Design review of the part built by this model. Coordinates are the model's own, in mm. A direction names the side the tool comes from. Round coordinates to 2 decimals unless told otherwise and drop trailing zeros. Write each loop counter-clockwise with the first axis right and the second up, starting at its lowest first coordinate (ties: lowest second). Pieces come first, ordered by that corner, then holes.
from build123d import *

# Parameters (mm, degrees)
F1_DEPTH = 4.064
F0_W     = 4.064
F0_H     = 4.064
F2_DEPTH = 4.064


# Not quite as in the source:
# - a feature names something its author has since deleted; it is built from what else it names


with BuildPart() as f1:
    # F0 (on Top) → F1 (new body)
    with BuildSketch(Plane.XY):
        Polygon((31.75, 12.7), (31.75, 25.4), (-31.75, 25.4), (-31.75, 12.7), (-27.686, 12.7), (-27.686, -12.7), (-31.75, -12.7), (-31.75, -25.4), (-25.4, -25.4), (-25.4, -21.336), (25.4, -21.336), (25.4, -25.4), (31.75, -25.4), (31.75, -12.7), (27.686, -12.7), (27.686, 12.7), align=None)
    extrude(amount=F1_DEPTH)

    # F0 (on Top) → F2 (join)
    with BuildSketch(Plane.XY):
        Polygon((21.336, -25.4), (25.4, -25.4), (25.4, -21.336), (-25.4, -21.336), (-25.4, -25.4), (-21.336, -25.4), align=None)
        with Locations((23.368, -27.432)):
            Rectangle(F0_W, F0_H)
        with Locations((-23.368, -27.432)):
            Rectangle(F0_W, F0_H)
        Polygon((31.75, 12.7), (31.75, 25.4), (-31.75, 25.4), (-31.75, 12.7), (-27.686, 12.7), (-27.686, -12.7), (-31.75, -12.7), (-31.75, -25.4), (-25.4, -25.4), (-25.4, -21.336), (25.4, -21.336), (25.4, -25.4), (31.75, -25.4), (31.75, -12.7), (27.686, -12.7), (27.686, 12.7), align=None)
    extrude(amount=F2_DEPTH)


solid = f1.part
1) Add section B-B on x = -12.5. State the section outline as (y, z) points, and give its area (3 significant figures).
2) The part is to be moulded in two halves that separate along Y. For faces 1 (the face through (0, -2, 4.064)), 2 (the face through (30, -12.7, 2)), 3 (the face through (-23, -29.464, 2)), say which applies: pulls with the +Y half, pulls with the -Y half, needs draft (parallel to the pull), parting line crosses it, or undercut.
3) For line 1 along Y through (x, z) = (-26.5, 1.75); line 2 along Y through (x, z) = (-28, 1.2); line 3 along X through (y, z) = (-8, 2.55), list the stretches that pass through material, from the lowest coordinate up.
4) For P1, Ø2, axis at x = 30, z = 2.5, coming from the -Y side; P2, Ø1.2, axis at y = -27.5, z = 1.5, coming from the -X side; P3, Ø1.2, axis at y = -27.5, z = 3, coming from the +X side, all flat-tipped, find the tip position at first contact; note any pin that passes through.
5) Add section A-A on z = 2.2. State the section outline as (x, y) points.
6) Add section C-C on y = -1. State the section outline as (x, z) points.
7) For faces 4 (the face through (30, 12.7, 2)), 5 (the face through (-27.686, 0, 2)), 6 (the face through (25.4, -27, 2)), 7 (the face through (21.336, -27, 2)), 8 (the face through (-29, -25.4, 2)), list the 3-axis set-ups (+Z, -Z, +X, -X, +Y, -Y) from which the entire face can be reached by the end or side of a thin tool; tool diameter is ignored.
Computed:
1. outline: (-25.4, 0) - (25.4, 0) - (25.4, 4.06) - (-25.4, 4.06) - close
1. area: 206 mm2
2. face 1: needs draft
2. face 2: undercut
2. face 3: pulls with the -Y half
3. line 1: y = -25.4 to 25.4
3. line 2: y = -25.4 to -12.7, 12.7 to 25.4
3. line 3: x = -27.69 to 27.69
4. P1: stops at y = -25.4
4. P2: stops at x = -25.4
4. P3: stops at x = 25.4
5. outline: (-31.75, -25.4) - (-25.4, -25.4) - (-25.4, -29.46) - (-21.34, -29.46) - (-21.34, -25.4) - (21.34, -25.4) - (21.34, -29.46) - (25.4, -29.46) - (25.4, -25.4) - (31.75, -25.4) - (31.75, -12.7) - (27.69, -12.7) - (27.69, 12.7) - (31.75, 12.7) - (31.75, 25.4) - (-31.75, 25.4) - (-31.75, 12.7) - (-27.69, 12.7) - (-27.69, -12.7) - (-31.75, -12.7) - close
6. outline: (-27.69, 0) - (27.69, 0) - (27.69, 4.06) - (-27.69, 4.06) - close
7. face 4: +Z, -Z, +X
7. face 5: +Z, -Z, -X
7. face 6: +Z, -Z, +X, -Y
7. face 7: +Z, -Z, -Y
7. face 8: +Z, -Z, -X, -Y
